The listing builds one solid part. Answer for the finished solid, in the listing's coordinates (mm). Give positions to 0.01 mm unless a question says otherwise; leave off trailing zeros. Order: outer loops, then holes, each group sorted by start corner. A loop starts at its lowest first (then second) coordinate and runs counter-clockwise, first axis right, second up. Notation, with made-up numbers: (59, 43) - (82, 43) arc R19 ccw to (82, 63) - close; hole circle Ø7 at (71, 53). An arc over 180 degrees is marked (long way). Write each question's results on one line, items separated by ' | '. Start each with the question number.
1. Determine the mould class of faces 1 (the face through (-55.852, 0.79, -12.403)), 2 (the face through (-33.337, 1.234, -43.477)), 3 (the face through (-54, 2.5, 12)) for opening direction X: released by +X, released by -X, zero draft, split by the parting line, or undercut.
2. Section C-C (y = 0.65) is taken. Give the vertices of the cut face in (x, z) (1 decimal), and give its area (3 significant figures).
3. Section B-B (z = 0) is taken. Give the vertices of the cut face in (x, y), and give its area (3 significant figures).
4. A flat-ended cylindrical pin translates along its axis: pin 1 (1.5 mm diameter, centred on x = -35, y = 2, fed in from -Z). Find the tip coordinate at first contact, or state that the pin passes through.
5. Find the intervals of material crossed by L1, parallel to X at y = 1.25, z = 0; L2, parallel to X at y = 1.6, z = 0; L3, parallel to Z at x = 36, y = 1.1, in increasing order.
6. Section A-A (x = 0) is taken. Give the vertices of the cut face in (y, z), and give its area (3 significant figures).
from build123d import *

# Parameters (mm, degrees)
SKETCH1_R           = 57.2125
SKETCH1_R_2         = 54.7875
BOSS_EXTRUDE1_DEPTH = 2.5
CHAMFER1_SIZE       = 1
FILLET1_R           = 0.1


with BuildPart() as part:
    # Sketch1 → Boss-Extrude1 (new body)
    with BuildSketch(Plane(origin=(0, 0, 0), x_dir=(1, 0, 0), z_dir=(0, 1, 0))):
        with Locations(Location((0, 0, 0), (0, 0, 270))):
            Circle(SKETCH1_R)
        with Locations(Location((0, 0, 0), (0, 0, 270))):
            Circle(SKETCH1_R_2, mode=Mode.SUBTRACT)
    extrude(amount=BOSS_EXTRUDE1_DEPTH)

    # Chamfer1
    chamfer1_edges = [part.edges().sort_by_distance(p)[0] for p in [
        (0, 2.5, -57.2125),
    ]]
    chamfer(chamfer1_edges, length=CHAMFER1_SIZE)

    # Fillet1
    fillet1_edges = [part.edges().sort_by_distance(p)[0] for p in [
        (0, 0, -57.2125),
        (0, 0, -54.7875),
        (0, 2.5, -54.7875),
    ]]
    fillet(fillet1_edges, radius=FILLET1_R)


solid = part.part
Reported:
1) face 1: split by the parting line | face 2: undercut | face 3: zero draft
2) outline: circle Ø114.4 at (0, 0); hole circle Ø109.6 at (0, 0) | area: 853 mm²
3) outline: (-57.21, 0.1) arc R0.1 ccw to (-57.11, 0) - (-54.89, 0) arc R0.1 ccw to (-54.79, 0.1) - (-54.79, 2.4) arc R0.1 ccw to (-54.89, 2.5) - (-56.21, 2.5) - (-57.21, 1.5) - close; (54.79, 0.1) arc R0.1 ccw to (54.89, 0) - (57.11, 0) arc R0.1 ccw to (57.21, 0.1) - (57.21, 1.5) - (56.21, 2.5) - (54.89, 2.5) arc R0.1 ccw to (54.79, 2.4) - close | area: 11.1 mm²
4) pin 1: z = -45.68
5) L1: -57.21 to -54.79, 54.79 to 57.21 | L2: -57.11 to -54.79, 54.79 to 57.11 | L3: -44.47 to -41.3, 41.3 to 44.47
6) outline: (0, -57.11) arc R0.1 ccw to (0.1, -57.21) - (1.5, -57.21) - (2.5, -56.21) - (2.5, -54.89) arc R0.1 ccw to (2.4, -54.79) - (0.1, -54.79) arc R0.1 ccw to (0, -54.89) - close; (0, 54.89) arc R0.1 ccw to (0.1, 54.79) - (2.4, 54.79) arc R0.1 ccw to (2.5, 54.89) - (2.5, 56.21) - (1.5, 57.21) - (0.1, 57.21) arc R0.1 ccw to (0, 57.11) - close | area: 11.1 mm²
